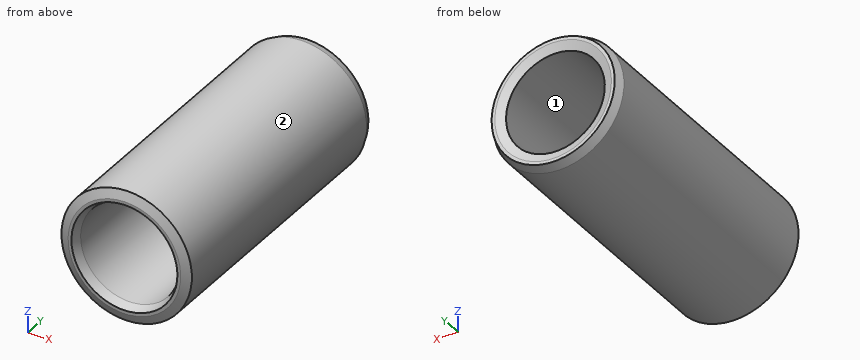
```python
from build123d import *
from OCP.BRepFilletAPI import BRepFilletAPI_MakeChamfer

# Parameters (mm, degrees)
SKETCH1_R           = 17.5
BOSS_EXTRUDE1_DEPTH = 78.797027
SKETCH2_R           = 13.247345897
CUT_EXTRUDE1_DEPTH  = 83.592199777
CHAMFER1_SIZE       = 2.391465
CHAMFER1_SIZE2      = 0.972886


with BuildPart() as part:
    # Sketch1 → Boss-Extrude1 (new body)
    with BuildSketch(Plane(origin=(0, 0, 0), x_dir=(1, 0, 0), z_dir=(0, 1, 0))):
        with Locations(Location((0, 0, 0), (0, 0, 270))):
            Circle(SKETCH1_R)
    extrude(amount=BOSS_EXTRUDE1_DEPTH)

    # Sketch2 → Cut-Extrude1 (cut, through all)
    with BuildSketch(Plane(origin=(0, 0, 0), x_dir=(1, 0, 0), z_dir=(0, 1, 0))):
        with Locations(Location((0, 0, 0), (0, 0, 270))):
            Circle(SKETCH2_R)
    extrude(amount=CUT_EXTRUDE1_DEPTH, mode=Mode.SUBTRACT)

    # Chamfer1: one chamfer whose edges measure the first distance from different faces: ONE call of the kernel's chamfer builder (chamfer() names one face for all edges)
    chamfer1_edges_1 = [part.edges().sort_by_distance(p)[0] for p in [
        (0, 0, -17.5),
    ]]
    chamfer1_side_1 = [part.faces().sort_by_distance(p)[0] for p in [
        (0, 0, -17.005025253),
    ]]
    chamfer1_edges_2 = [part.edges().sort_by_distance(p)[0] for p in [
        (0, 78.797027, -17.5),
    ]]
    chamfer1_side_2 = [part.faces().sort_by_distance(p)[0] for p in [
        (0, 39.3985135, -17.5),
    ]]
    chamfer1_edges_3 = [part.edges().sort_by_distance(p)[0] for p in [
        (0, 0, -13.247345897),
    ]]
    chamfer1_side_3 = [part.faces().sort_by_distance(p)[0] for p in [
        (0, 39.3985135, -13.247345897),
    ]]
    chamfer1_edges_4 = [part.edges().sort_by_distance(p)[0] for p in [
        (0, 78.797027, -13.247345897),
    ]]
    chamfer1_side_4 = [part.faces().sort_by_distance(p)[0] for p in [
        (0, 78.797027, -17.005025253),
    ]]
    chamfer1 = BRepFilletAPI_MakeChamfer(part.part.solid().wrapped)
    for e in chamfer1_edges_1:
        chamfer1.Add(CHAMFER1_SIZE, CHAMFER1_SIZE2, e.wrapped, chamfer1_side_1[0].wrapped)  # the first distance lies on this face
    for e in chamfer1_edges_2:
        chamfer1.Add(CHAMFER1_SIZE, CHAMFER1_SIZE2, e.wrapped, chamfer1_side_2[0].wrapped)  # the first distance lies on this face
    for e in chamfer1_edges_3:
        chamfer1.Add(CHAMFER1_SIZE, CHAMFER1_SIZE2, e.wrapped, chamfer1_side_3[0].wrapped)  # the first distance lies on this face
    for e in chamfer1_edges_4:
        chamfer1.Add(CHAMFER1_SIZE, CHAMFER1_SIZE2, e.wrapped, chamfer1_side_4[0].wrapped)  # the first distance lies on this face
    add(Compound.cast(chamfer1.Shape()), mode=Mode.REPLACE)


solid = part.part
```
Design review of the part built by this model. Coordinates are the model's own, in mm. Face numbers are marked on the shaded views. Give positions to 0.01 mm unless a question says otherwise; leave off trailing zeros. Loops run counter-clockwise (first coordinate to the right, second up) from the corner with the lowest first, then second, coordinate; pieces in that order, holes last. Notation, with made-up numbers: (19, 7.25) -> (25, 7.25) arc R14 ccw to (25, 12.25) -> close; hole circle Ø4 at (61.25, -28). An arc over 180 degrees is marked (long way). Write each question's results on one line, items separated by ' | '.
Q1. Take a section at C-C, the plane y = 28. Write out the cut boundary in (x, z), plus the area to 3 significant figures.
Reply:
outline: circle Ø35 at (0, 0); hole circle Ø26.49 at (0, 0) | area: 411 mm²
Q2. For pin 1 Ø5 at (y, z) = (70.5, -13) entering from -X; pin 2 Ø10 at (y, z) = (32.5, 10) entering from -X; pin 3 Ø4 at (x, z) = (10.5, 7) entering from -Y; pin 4 Ø1 at (x, y) = (1, 58) entering from -Z, all flat-tipped, find the tip position at first contact; note any pin that passes through.
Reply:
pin 1: stops at x = -14 | pin 2: stops at x = -16.77 | pin 3: stops at y = 0 | pin 4: stops at z = -17.49
Q3. Wall thickness on L1, parallel to Z at x = -11, y = 34; L2, parallel to X at y = 31.5, z = 0; L3, parallel to X at y = 67, z = 12: over which ranges is each line inside the solid? List them lowest first.
Reply:
L1: z = -13.61 to -7.38, 7.38 to 13.61 | L2: x = -17.5 to -13.25, 13.25 to 17.5 | L3: x = -12.74 to -5.61, 5.61 to 12.74
Q4. Take a section at B-B, the plane z = 0. Write out the cut boundary in (x, y).
Reply:
outline: (-17.5, 0.97) -> (-15.11, 0) -> (-14.22, 0) -> (-13.25, 2.39) -> (-13.25, 77.82) -> (-15.64, 78.8) -> (-16.53, 78.8) -> (-17.5, 76.41) -> close; (13.25, 2.39) -> (14.22, 0) -> (15.11, 0) -> (17.5, 0.97) -> (17.5, 76.41) -> (16.53, 78.8) -> (15.64, 78.8) -> (13.25, 77.82) -> close
Q5. The part is to be moulded in two halves that separate along X. For the marked faces 1 and 2, say which applies: +X half, -X half, draft (parallel to the pull), parting line (faces both ways), or undercut.
Reply:
face 1: undercut | face 2: parting line
Q6. Take a section at A-A, the plane x = 0. Write out the cut boundary in (y, z).
Reply:
outline: (0, -15.11) -> (0.97, -17.5) -> (76.41, -17.5) -> (78.8, -16.53) -> (78.8, -15.64) -> (77.82, -13.25) -> (2.39, -13.25) -> (0, -14.22) -> close; (0, 14.22) -> (2.39, 13.25) -> (77.82, 13.25) -> (78.8, 15.64) -> (78.8, 16.53) -> (76.41, 17.5) -> (0.97, 17.5) -> (0, 15.11) -> close
